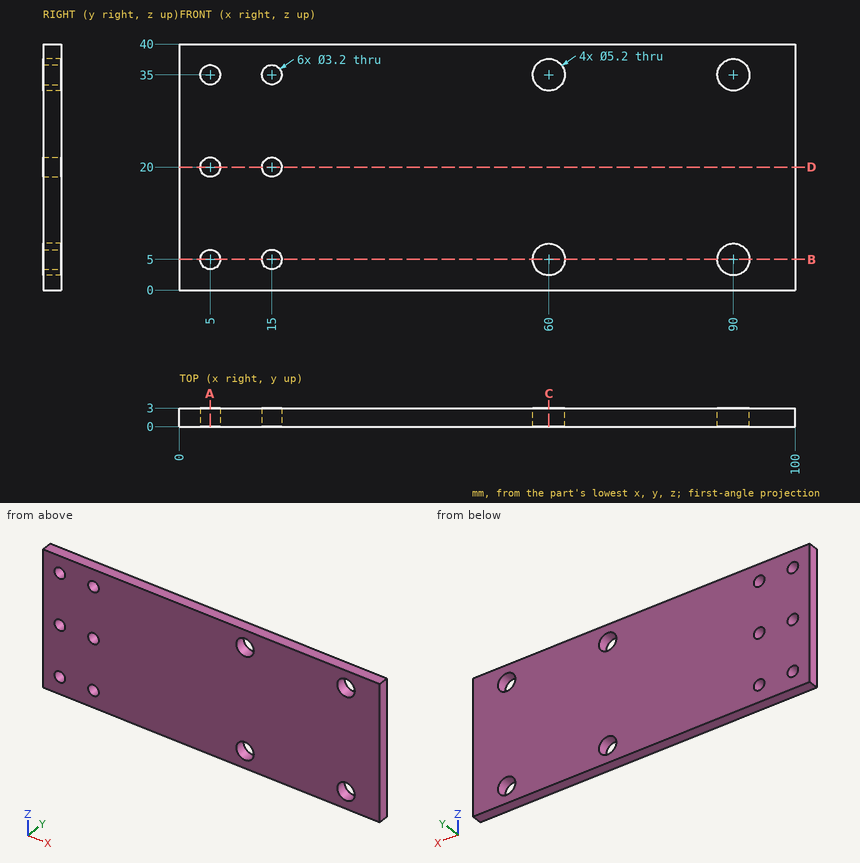
The figure shows three views and two pictorial views of one solid part (mm, origin at its lowest corner). Answer the questions. Round coordinates to 2 decimals unless told otherwise and drop trailing zeros. Order: outer loops, then holes, each group sorted by start corner. A loop starts at its lowest first (then second) coordinate and runs counter-clockwise, first axis right, second up. Notation, with made-up numbers: (-26.5, 42.25) - (27.5, 42.25) arc R23 cw to (27.5, 61.25) - close; hole circle Ø3 at (70, 9). An arc over 180 degrees is marked (long way). Write item = value, one per line. Start each with the question number.
1) Section B-B, the plane z = 5 is taken. Write down the section's boundary in (x, y), plus the area to 3 significant figures.
2) Section C-C, the plane x = 60 is taken. Write down the section's boundary in (y, z).
3) Given pin 1 (3.5 mm diameter, centred on x = 15, z = 5, fed in from -Y); pin 2 (4 mm diameter, centred on x = 90, z = 5, fed in from +Y), each flat-ended and moving along its own axis, determine where each tip first touches the part or whether it passes through.
4) Section A-A, the plane x = 5 is taken. Write down the section's boundary in (y, z).
5) Straight lines are drawn through the part: L1, parallel to X at y = 0.9, z = 35; L2, parallel to X at y = 1.8, z = 20; L3, parallel to Z at x = 6, y = 2.85. For each, find the intervals that lie inside material, in ascending order.
6) Section D-D, the plane z = 20 is taken. Write down the section's boundary in (x, y).
Results list:
q1.outline = (0, 0) - (3.4, 0) - (3.4, 3) - (0, 3) - close; (6.6, 0) - (13.4, 0) - (13.4, 3) - (6.6, 3) - close; (16.6, 0) - (57.4, 0) - (57.4, 3) - (16.6, 3) - close; (62.6, 0) - (87.4, 0) - (87.4, 3) - (62.6, 3) - close; (92.6, 0) - (100, 0) - (100, 3) - (92.6, 3) - close
q1.area = 250 mm^2
q2.outline = (0, 0) - (3, 0) - (3, 2.4) - (0, 2.4) - close; (0, 7.6) - (3, 7.6) - (3, 32.4) - (0, 32.4) - close; (0, 37.6) - (3, 37.6) - (3, 40) - (0, 40) - close
q3.pin_1 = 0
q3.pin_2 = through
q4.outline = (0, 0) - (3, 0) - (3, 3.4) - (0, 3.4) - close; (0, 6.6) - (3, 6.6) - (3, 18.4) - (0, 18.4) - close; (0, 21.6) - (3, 21.6) - (3, 33.4) - (0, 33.4) - close; (0, 36.6) - (3, 36.6) - (3, 40) - (0, 40) - close
q5.L1 = 0 to 3.4, 6.6 to 13.4, 16.6 to 57.4, 62.6 to 87.4, 92.6 to 100
q5.L2 = 0 to 3.4, 6.6 to 13.4, 16.6 to 100
q5.L3 = 0 to 3.75, 6.25 to 18.75, 21.25 to 33.75, 36.25 to 40
q6.outline = (0, 0) - (3.4, 0) - (3.4, 3) - (0, 3) - close; (6.6, 0) - (13.4, 0) - (13.4, 3) - (6.6, 3) - close; (16.6, 0) - (100, 0) - (100, 3) - (16.6, 3) - close
